Part print with two shaded views. Sizes in mm from the minimum x, y, z corner. Give positions to 0.01 mm unless a question says otherwise; leave off trailing zeros. Order: outer loops, then holes, each group sorted by start corner. A loop starts at its lowest first (then second) coordinate and runs counter-clockwise, first axis right, second up.
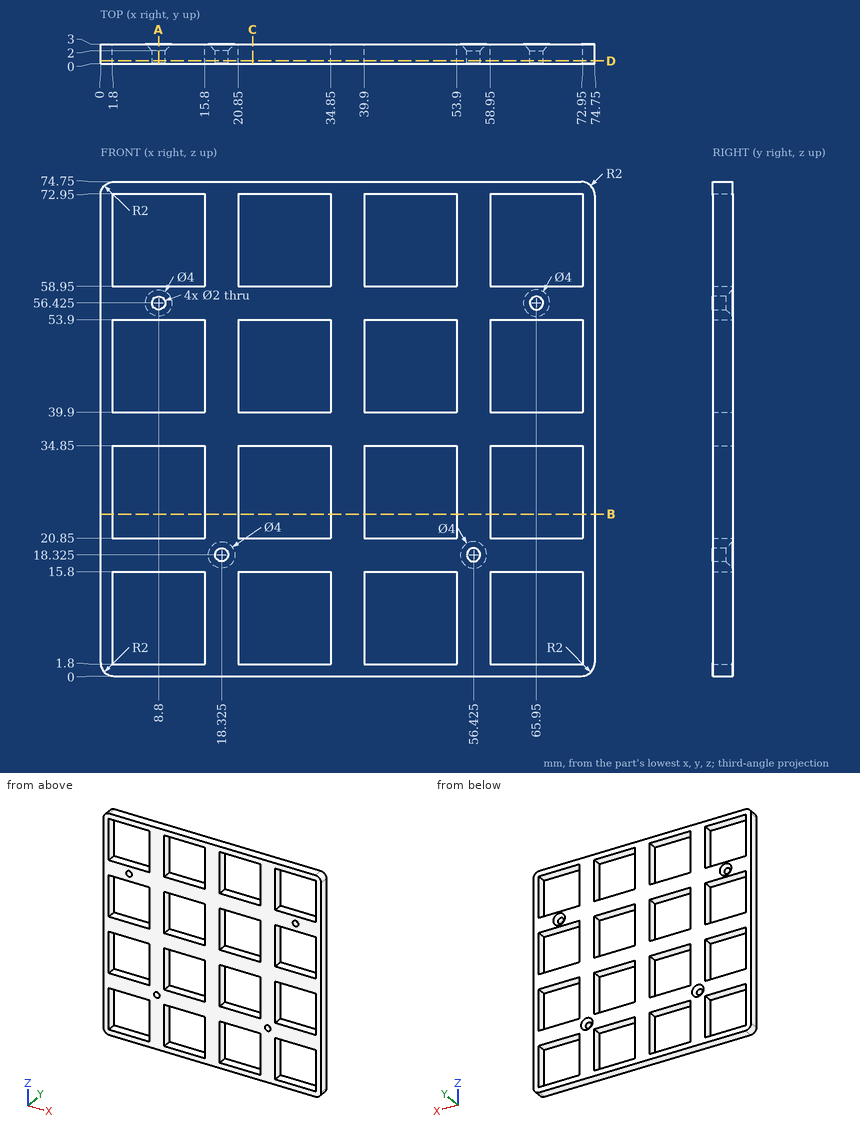
Item 1: Slice it at A-A (x = 8.8). Give the cut face in (y, z) (3 decimals), and give its area (4 significant figures).
Item 2: Drop a flat-ended pin along its axis: pin 1 Ø10 at (x, z) = (47, 47) entering from -Y. Give the stop position or say it passes through.
Item 3: Slice it at B-B (z = 24.5). Give the cut face in (x, y).
Item 4: Slice it at C-C (x = 23). Give the cut face in (y, z).
Item 5: Wall check: L1, parallel to Z at x = 34, y = 0.6; L2, parallel to Z at x = 9, y = 1.7. Give the ranges that are in metal, low to high.
Item 6: Slice it at D-D (y = 0.45). State how many separate pieces and enclosed holes the cut face has, and give its area (3 significant figures).
A:
1. outline: (0, 0) - (3, 0) - (3, 1.8) - (0, 1.8) - close; (0, 15.8) - (3, 15.8) - (3, 20.85) - (0, 20.85) - close; (0, 34.85) - (3, 34.85) - (3, 39.9) - (0, 39.9) - close; (0, 53.9) - (3, 53.9) - (3, 54.425) - (2, 55.425) - (0, 55.425) - close; (0, 57.425) - (2, 57.425) - (3, 58.425) - (3, 58.95) - (0, 58.95) - close; (0, 72.95) - (3, 72.95) - (3, 74.75) - (0, 74.75) - close
1. area: 49.25 mm2
2. pin 1: passes through
3. outline: (0, 0) - (1.8, 0) - (1.8, 3) - (0, 3) - close; (15.8, 0) - (20.85, 0) - (20.85, 3) - (15.8, 3) - close; (34.85, 0) - (39.9, 0) - (39.9, 3) - (34.85, 3) - close; (53.9, 0) - (58.95, 0) - (58.95, 3) - (53.9, 3) - close; (72.95, 0) - (74.75, 0) - (74.75, 3) - (72.95, 3) - close
4. outline: (0, 0) - (3, 0) - (3, 1.8) - (0, 1.8) - close; (0, 15.8) - (3, 15.8) - (3, 20.85) - (0, 20.85) - close; (0, 34.85) - (3, 34.85) - (3, 39.9) - (0, 39.9) - close; (0, 53.9) - (3, 53.9) - (3, 58.95) - (0, 58.95) - close; (0, 72.95) - (3, 72.95) - (3, 74.75) - (0, 74.75) - close
5. L1: z = 0 to 1.8, 15.8 to 20.85, 34.85 to 39.9, 53.9 to 58.95, 72.95 to 74.75
5. L2: z = 0 to 1.8, 15.8 to 20.85, 34.85 to 39.9, 53.9 to 55.45, 57.4 to 58.95, 72.95 to 74.75
6. separate pieces: 1
6. enclosed holes: 20
6. area: 2,440 mm2
